Verification items for this drawing (mm, ordinates from the low corner). A direction names the side the tool comes from. Coordinates: 2 decimals unless noted, no trailing zeros. Loops run counter-clockwise (first coordinate to the right, second up) from the corner with the lowest first, then second, coordinate; pieces in that order, holes last. Notation, with made-up numbers: M -22,82.25 L 34,82.25 A14 ccw 34,87.25 Z; hole C 78.25,78.25 d2. An arc over 180 degrees is marked long. Return JSON: item names as keys, results as strings.
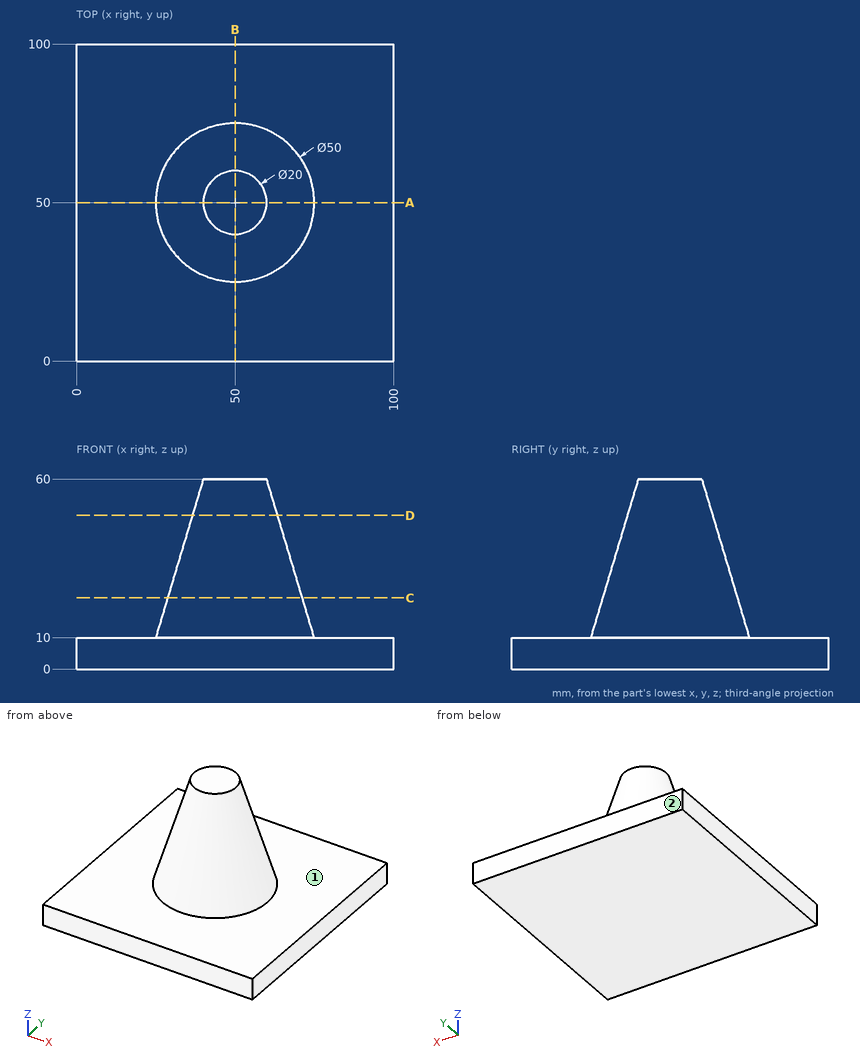
1) Section check D-D on z = 48.5. Record the cut outline in (x, y), then the cut area to 3 significant figures.
Answers:
{"outline": "C 50,50 d26.9", "area": "568 mm²"}
2) Scan lines: line 1 along Z through (x, y) = (92, 54); line 2 along Y through (x, z) = (61.5, 51); line 3 along X through (y, z) = (44.5, 41). Record each from-to range of solid material in increasing order. Write a range as [from, to].
Answers:
{"line 1": "[0, 10]", "line 2": "[44.61, 55.39]", "line 3": "[35.29, 64.71]"}
3) Section check C-C on z = 22.5. Record the cut outline in (x, y), then the cut area to 3 significant figures.
Answers:
{"outline": "C 50,50 d42.5", "area": "1,420 mm²"}
4) Section check A-A on y = 50. Record the cut outline in (x, z), then the cut area to 3 significant figures.
Answers:
{"outline": "M 0,0 L 100,0 L 100,10 L 75,10 L 60,60 L 40,60 L 25,10 L 0,10 Z", "area": "2,750 mm²"}
5) Set-up check for the marked faces 1 and 2: record each of +Z, -Z, +X, -X, +Y, -Y from which the full face is reachable in a straight line by a thin tool's end or side.
Answers:
{"face 1": "+Z", "face 2": "+Z, -Z, +X, -X, +Y"}
6) Go/stop test with flat-tipped pins: pin 1 Ø8 at (y, z) = (54.5, 24) entering from -X; pin 2 Ø5 at (y, z) = (75, 20) entering from +X; pin 3 Ø5 at (y, z) = (64, 18) entering from -X; pin 4 Ø4 at (x, z) = (39.5, 29) entering from +Y. Record where each tip stops, or that it passes through.
Answers:
{"pin 1": "x = 28.29", "pin 2": "through", "pin 3": "x = 30.31", "pin 4": "y = 67.53"}
